Geometry: final body of the model. Coordinates: model frame, mm. A direction names the side the tool comes from. Coordinates: 2 decimals unless noted, no trailing zeros. Write each loop counter-clockwise with the first axis right and the second up, starting at its lowest first coordinate (ties: lowest second). Pieces come first, ordered by that corner, then holes.
from build123d import *

# Parameters (mm, degrees)
SKETCH_1_W          = 100
SKETCH_1_H          = 50
EXTRUDE_1_DEPTH     = 10
EXTRUDE_START       = -10
EXTRUDE_2_DEPTH     = 20
SKETCH_3_R          = 12
CUT_EXTRUDE_1_DEPTH = 101
SKETCH_4_R          = 5
CUT_EXTRUDE_2_DEPTH = 86.732140997


# Read off the part's stored shape, not the designer's step: 凸台-拉伸2
with BuildPart() as part:
    # 草图1 → 凸台-拉伸1 (new body)
    with BuildSketch(Plane.XY):
        Rectangle(SKETCH_1_W, SKETCH_1_H)
    extrude(amount=EXTRUDE_1_DEPTH)

    # 凸台-拉伸2 outline → 凸台-拉伸2 (add)
    with BuildSketch(Plane(origin=(0, 0, 0), x_dir=(1, 0, 0), z_dir=(0, 1, 0)).offset(EXTRUDE_START)):
        with BuildLine():
            Line((-25, -10), (-25, -40))
            ThreePointArc((-25, -40), (0, -65), (25, -40))
            Line((25, -40), (25, -10))
            Line((25, -10), (-25, -10))
        make_face()
    extrude(amount=EXTRUDE_2_DEPTH)

    # 草图3 → 切除-拉伸1 (cut, symmetric)
    with BuildSketch(Plane(origin=(0, 0, 0), x_dir=(1, 0, 0), z_dir=(0, 1, 0))):
        with Locations(Location((0, -40, 0), (0, 0, 270))):
            Circle(SKETCH_3_R)
    extrude(amount=CUT_EXTRUDE_1_DEPTH, both=True, mode=Mode.SUBTRACT)

    # 草图4 → 切除-拉伸2 (cut, through all)
    with BuildSketch(Plane.XY):
        with Locations((-38, 0)):
            Circle(SKETCH_4_R)
        with Locations((38, 0)):
            Circle(SKETCH_4_R)
    extrude(amount=CUT_EXTRUDE_2_DEPTH, mode=Mode.SUBTRACT)


solid = part.part
Item 1: Section B-B, the plane z = 38. Output: boundary loops of the cut face in (x, y), plus the area to 3 significant figures.
Derived:
outline: (-25, -10) - (-11.83, -10) - (-11.83, 10) - (-25, 10) - close; (11.83, -10) - (25, -10) - (25, 10) - (11.83, 10) - close
area: 527 mm2
Item 2: Set-up query: faces 1 (the flat face through (25, 0, 25)), 2 (the flat face through (-25, 0, 25)), 3 (the flat face through (0, 10, 25)). Return all of +Z, -Z, +X, -X, +Y, -Y with unobstructed straight access to the full face (end or side cutting, diameter ignored); none if empty.
Derived:
face 1: +Z, +X, +Y, -Y
face 2: +Z, -X, +Y, -Y
face 3: +Z, +X, -X, +Y
Item 3: Section C-C, the plane x = 0. Output: boundary loops of the cut face in (y, z), plus the area to 3 significant figures.
Derived:
outline: (-25, 0) - (25, 0) - (25, 10) - (10, 10) - (10, 28) - (-10, 28) - (-10, 10) - (-25, 10) - close; (-10, 52) - (10, 52) - (10, 65) - (-10, 65) - close
area: 1,120 mm2
Item 4: Section D-D, the plane y = -13.5. Output: boundary loops of the cut face in (x, z).
Derived:
outline: (-50, 0) - (50, 0) - (50, 10) - (-50, 10) - close
Item 5: Pull-direction query (Y, two-part tool) for faces 4 (the cylindrical face through (33, 0, 5)), 5 (the cylindrical face through (-4.596, 0.14, 51.085)), 6 (the flat face through (0, -10, 25)), 7 (the cylindrical face through (-43, 0, 5)); classes: released by +Y, released by -Y, zero draft, split by the parting line, or undercut.
Derived:
face 4: undercut
face 5: zero draft
face 6: released by -Y
face 7: undercut
Item 6: Material intervals for probe 1 along X at (y, z) = (0, 4.5); probe 2 along Y at (x, z) = (-38, 6); probe 3 along X at (y, z) = (0.75, 40), sorted ascending.
Derived:
probe 1: x = -50 to -43, -33 to 33, 43 to 50
probe 2: y = -25 to -5, 5 to 25
probe 3: x = -25 to -12, 12 to 25
Item 7: Pin query (flat end, axial travel): pin 1 (3 mm diameter, centred on x = -27.5, z = 12.5, fed in from -Y); pin 2 (1.5 mm diameter, centred on x = -20.5, z = 38.5, fed in from -Y); pin 3 (16 mm diameter, centred on y = 1.5, z = 19, fed in from -X); pin 4 (10 mm diameter, centred on y = 1.5, z = 22.5, fed in from +X). Return the tip coordinate at first contact, or that it passes through.
Derived:
pin 1: passes through
pin 2: stops at y = -10
pin 3: stops at x = -25
pin 4: stops at x = 25
Item 8: Section A-A, the plane x = 38. Output: boundary loops of the cut face in (y, z).
Derived:
outline: (-25, 0) - (-5, 0) - (-5, 10) - (-25, 10) - close; (5, 0) - (25, 0) - (25, 10) - (5, 10) - close
